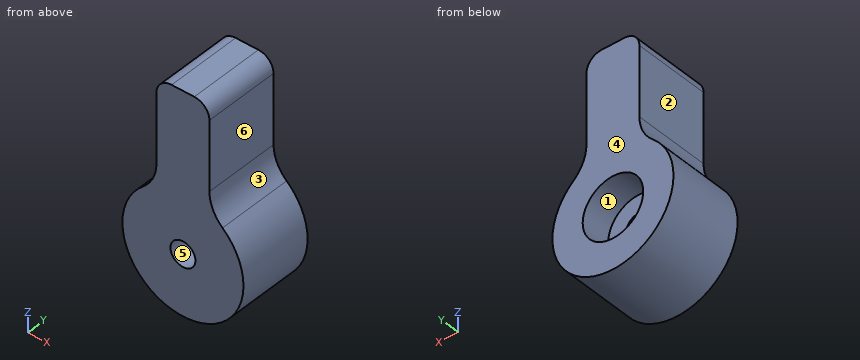
from build123d import *

# Parameters (mm, degrees)
EXTRUDE_1_DEPTH     = 10
FILLET_1_R          = 2
FILLET_2_R          = 5
SKETCH_4_R          = 4
CUT_EXTRUDE_1_DEPTH = 4
M4X0_71_D           = 3.3


with BuildPart() as part:
    # Эскиз1 → Бобышка-Вытянуть1 (new body)
    with BuildSketch(Plane(origin=(0, 0, 0), x_dir=(1, 0, 0), z_dir=(0, 1, 0))):
        with BuildLine():
            Line((-3.5, -7.193747285), (-3.5, -21))
            Line((-3.5, -21), (3.5, -21))
            Line((3.5, -21), (3.5, -7.193747285))
            ThreePointArc((3.5, -7.193747285), (0, 8), (-3.5, -7.193747285))
        make_face()
    extrude(amount=EXTRUDE_1_DEPTH)

    # Скругление1
    fillet_1_edges = [part.edges().sort_by_distance(p)[0] for p in [
        (3.5, 5, 21),
        (-3.5, 5, 21),
    ]]
    fillet(fillet_1_edges, radius=FILLET_1_R)

    # Скругление2
    fillet_2_edges = [part.edges().sort_by_distance(p)[0] for p in [
        (-3.5, 5, 7.193747285),
        (3.5, 5, 7.193747285),
    ]]
    fillet(fillet_2_edges, radius=FILLET_2_R)

    # Эскиз4 → Вырез-Вытянуть1 (cut)
    with BuildSketch(Plane(origin=(0, 10, 0), x_dir=(1, 0, 0), z_dir=(0, 1, 0))):
        Circle(SKETCH_4_R)
    extrude(amount=-CUT_EXTRUDE_1_DEPTH, mode=Mode.SUBTRACT)

    # Отверстие обработанное метчиком M4x0.71 (through all)
    with Locations(Plane(origin=(0, 6, 0), x_dir=(1, 0, 0), z_dir=(0, 1, 0))):
        with Locations((0, 0)):
            Hole(M4X0_71_D / 2)


solid = part.part
CAD build for the part. Positions are in the model's coordinates, mm. Face numbers are marked on the shaded views. A direction names the side the tool comes from. Round coordinates to 2 decimals unless told otherwise and drop trailing zeros. Loops run counter-clockwise (first coordinate to the right, second up) from the corner with the lowest first, then second, coordinate; pieces in that order, holes last. Notation, with made-up numbers: (78, 48.5) - (134, 48.5) arc R30 ccw to (134, 76.5) - close; hole circle Ø9 at (-13.5, -36). An arc over 180 degrees is marked (long way). Put each result on its own line as item: value.
1. Pin check, flat tips, straight feed: P1, Ø3, axis at y = 6, z = -1, coming from the -X side; P2, Ø2.5, axis at x = 0, z = -1.5, coming from the +Y side; P3, Ø2.5, axis at y = 4.5, z = 15.5, coming from the +X side. Stop position of each tip, or through.
Geometry check:
P1: x = -8
P2: y = 6
P3: x = 3.5
2. Slice it at D-D on y = 8. List the corners of the cut face in (x, z), and give its area (3 significant figures).
Geometry check:
outline: (-5.23, 6.05) arc R8 ccw (long way) to (5.23, 6.05) arc R5 cw to (3.5, 9.84) - (3.5, 19) arc R2 ccw to (1.5, 21) - (-1.5, 21) arc R2 ccw to (-3.5, 19) - (-3.5, 9.84) arc R5 cw to start; hole circle Ø8 at (0, 0)
area: 244 mm²
3. Wall check: line 1 (X direction, y = 7.15, z = 0); line 2 (Y direction, x = -1.75, z = 0); line 3 (Z direction, x = 3, y = 7). Give the ranges that are in metal, low to high.
Geometry check:
line 1: -8 to -4, 4 to 8
line 2: 0 to 6
line 3: -7.42 to -2.65, 2.65 to 20.32
4. 3-axis set-ups, long thin cutter, end or side, ignore diameter. For the marked faces 5 and 6: which of +Z, -Z, +X, -X, +Y, -Y reach the whole face in a straight line?
Geometry check:
face 5: +Y, -Y
face 6: +Z, +X, +Y, -Y
5. Two-plate mould, pull along X, no slides. Class the marked faces 1, 2, 3 and 4: released by +X, released by -X, zero draft, split by the parting line, or undercut.
Geometry check:
face 1: undercut
face 2: released by -X
face 3: released by +X
face 4: zero draft
6. Slice it at C-C on y = 3. List the corners of the cut face in (x, z).
Geometry check:
outline: (-5.23, 6.05) arc R8 ccw (long way) to (5.23, 6.05) arc R5 cw to (3.5, 9.84) - (3.5, 19) arc R2 ccw to (1.5, 21) - (-1.5, 21) arc R2 ccw to (-3.5, 19) - (-3.5, 9.84) arc R5 cw to start; hole circle Ø3.3 at (0, 0)
7. Slice it at B-B on x = 0. List the corners of the cut face in (y, z).
Geometry check:
outline: (0, -8) - (10, -8) - (10, -4) - (6, -4) - (6, -1.65) - (0, -1.65) - close; (0, 1.65) - (6, 1.65) - (6, 4) - (10, 4) - (10, 21) - (0, 21) - close
8. Slice it at A-A on z = 0. List the corners of the cut face in (x, y).
Geometry check:
outline: (-8, 0) - (-1.65, 0) - (-1.65, 6) - (-4, 6) - (-4, 10) - (-8, 10) - close; (1.65, 0) - (8, 0) - (8, 10) - (4, 10) - (4, 6) - (1.65, 6) - close
